Design review of the part built by this model. Coordinates are the model's own, in mm. A direction names the side the tool comes from. Give positions to 0.01 mm unless a question says otherwise; leave off trailing zeros. Order: outer loops, then holes, each group sorted by start corner. A loop starts at its lowest first (then second) coordinate and runs counter-clockwise, first axis right, second up. Notation, with made-up numbers: (34.5, 36.5) -> (83.5, 36.5) arc R15 ccw to (83.5, 53.5) -> close; hole circle Ø9 at (-2, 56). An arc over 180 degrees is marked (long way). One line per item, written item: value.
from build123d import *

# Parameters (mm, degrees)
F0_W      = 76
F0_H      = 68
F0_W_2    = 56
F0_H_2    = 25
F0_W_3    = 6
F0_H_3    = 30
F1_DEPTH  = 2
F2_W      = 80
F2_H      = 142
F3_DEPTH  = 2
F4_R      = 1.99999
F6_DEPTH  = 4
F7_R      = 4
F8_R      = 2
F9_W      = 2
F9_H      = 4
F10_DEPTH = 100


# Not quite as in the source:
# - a fillet or chamfer is up to 0.001 mm smaller than in the source, because OpenCascade refuses the exact size


with BuildPart() as f1:
    # F0 (on Front) → F1 (new body)
    with BuildSketch(Plane.XZ):
        with Locations((-2, -1)):
            Rectangle(F0_W, F0_H)
        with Locations((-2, -19.5)):
            Rectangle(F0_W_2, F0_H_2, mode=Mode.SUBTRACT)
        with Locations((-32, 12)):
            Rectangle(F0_W_3, F0_H_3, mode=Mode.SUBTRACT)
        with Locations((-20, 12)):
            Rectangle(F0_W_3, F0_H_3, mode=Mode.SUBTRACT)
        with Locations((-8, 12)):
            Rectangle(F0_W_3, F0_H_3, mode=Mode.SUBTRACT)
        with Locations((4, 12)):
            Rectangle(F0_W_3, F0_H_3, mode=Mode.SUBTRACT)
        with Locations((16, 12)):
            Rectangle(F0_W_3, F0_H_3, mode=Mode.SUBTRACT)
        with Locations((28, 12)):
            Rectangle(F0_W_3, F0_H_3, mode=Mode.SUBTRACT)
    extrude(amount=F1_DEPTH)

    # F2 (on face) → F3 (join)
    with BuildSketch(Plane.XY.offset(33)):
        with Locations((-2, 69)):
            Rectangle(F2_W, F2_H)
    extrude(amount=F3_DEPTH)

    # F4 (radius 2 in the source; OpenCascade refuses exactly that, so slightly less here)
    f4_edges = [f1.edges().sort_by_distance(p)[0] for p in [
        (38, 69, 35),
        (-42, 69, 35),
    ]]
    fillet(f4_edges, radius=F4_R)

    # F5 (on face) → F6 (join)
    with BuildSketch(Plane(origin=(0, 0, 33), x_dir=(1, 0, 0), z_dir=(0, 0, -1))):
        Polygon((-38, 0), (-40, 0), (-40, -138), (36, -138), (36, 0), (34, 0), (34, -136), (-38, -136), align=None)
    extrude(amount=F6_DEPTH)

    # F7
    f7_edges = [f1.edges().sort_by_distance(p)[0] for p in [
        (-30, -1, -7),
        (26, -1, -7),
        (-30, -1, -32),
        (26, -1, -32),
    ]]
    fillet(f7_edges, radius=F7_R)

    # F8
    f8_edges = [f1.edges().sort_by_distance(p)[0] for p in [
        (-35, -1, 27),
        (-29, -1, 27),
        (-35, -1, -3),
        (-29, -1, -3),
        (-23, -1, 27),
        (-17, -1, 27),
        (-23, -1, -3),
        (-17, -1, -3),
        (-11, -1, -3),
        (-11, -1, 27),
        (-5, -1, 27),
        (-5, -1, -3),
        (1, -1, -3),
        (7, -1, -3),
        (7, -1, 27),
        (1, -1, 27),
        (13, -1, 27),
        (19, -1, 27),
        (19, -1, -3),
        (13, -1, -3),
        (25, -1, -3),
        (31, -1, -3),
        (25, -1, 27),
        (31, -1, 27),
    ]]
    fillet(f8_edges, radius=F8_R)

    # F9 (on face) → F10 (cut, symmetric)
    with BuildSketch(Plane(origin=(-40, 0, 0), x_dir=(0, -1, 0), z_dir=(-1, 0, 0))):
        with Locations((-117, 31)):
            Rectangle(F9_W, F9_H)
        with Locations((-21, 31)):
            Rectangle(F9_W, F9_H)
    extrude(amount=F10_DEPTH, both=True, mode=Mode.SUBTRACT)


solid = f1.part
Item 1: Draft analysis for pull direction X (two halves, no side actions). For faces 1 (the flat face through (-3, -2, 7)), 2 (the flat face through (36, -1, 14)), 3 (the flat face through (-38, 127, 31)), state which applies: pulls with the +X half, pulls with the -X half, needs draft (parallel to the pull), parting line crosses it, or undercut.
Returned:
face 1: needs draft
face 2: pulls with the +X half
face 3: undercut
Item 2: To check wall thickness, follow line 1 along X through (y, z) = (119, 32); line 2 along Y through (x, z) = (-37.5, 30); line 3 along Y through (x, z) = (-28.5, 1). State the ranges of each line that lie inside material, in increasing order. Write a range as from..to.
Returned:
line 1: -40..-38, 34..36
line 2: -2..0, 136..138
line 3: -2..0
Item 3: Add section A-A on z = -22.5. Give the boundary of the cut face in (x, y), plus the area to 3 significant figures.
Returned:
outline: (-40, -2) -> (-30, -2) -> (-30, 0) -> (-40, 0) -> close; (26, -2) -> (36, -2) -> (36, 0) -> (26, 0) -> close
area: 40.0 mm²
Item 4: Clearance check with flat-ended pins moving along their axes: P1, Ø10, axis at x = -15, y = 126, coming from the -Z side; P2, Ø1, axis at x = -39, z = 31, coming from the +Y side; P3, Ø2, axis at y = 125.5, z = 30.5, coming from the -X side. State where each tip first meets the part, or that it passes through.
Returned:
P1: z = 33
P2: y = 138
P3: x = -40
Item 5: Add section B-B on x = 9. Give the boundary of the cut face in (y, z).
Returned:
outline: (-2, -35) -> (0, -35) -> (0, -32) -> (-2, -32) -> close; (-2, -7) -> (0, -7) -> (0, 33) -> (136, 33) -> (136, 29) -> (138, 29) -> (138, 33) -> (140, 33) -> (140, 35) -> (-2, 35) -> close
Item 6: Machinability: for faces 4 (the cylindrical face through (-28.859, -1.014, -30.797)), 5 (the flat face through (-38, 10, 31)), 6 (the flat face through (36, 70, 31)), 7 (the flat face through (-40, 68, 31)), which of the approach directions +Z, -Z, +X, -X, +Y, -Y give a long, thin tool a straight path to every point of the face, cutting with its end or side? Answer none if there is none.
Returned:
face 4: +Y, -Y
face 5: -Z
face 6: -Z, +X, +Y, -Y
face 7: -Z, -X, +Y, -Y
Item 7: Add section C-C on z = 15. Give the boundary of the cut face in (x, y).
Returned:
outline: (-40, -2) -> (-35, -2) -> (-35, 0) -> (-40, 0) -> close; (-29, -2) -> (-23, -2) -> (-23, 0) -> (-29, 0) -> close; (-17, -2) -> (-11, -2) -> (-11, 0) -> (-17, 0) -> close; (-5, -2) -> (1, -2) -> (1, 0) -> (-5, 0) -> close; (7, -2) -> (13, -2) -> (13, 0) -> (7, 0) -> close; (19, -2) -> (25, -2) -> (25, 0) -> (19, 0) -> close; (31, -2) -> (36, -2) -> (36, 0) -> (31, 0) -> close
